```python
from build123d import *

# Parameters (mm, degrees)
SKETCH1_R                = 41.9034
SKETCH1_R_2              = 39.9034
BOSS_EXTRUDE1_DEPTH      = 57.15
BOSS_EXTRUDE2_REACH      = 137.075
BOSS_EXTRUDE2_END_RADIUS = 41.9034
SKETCH4_W                = 6.35
SKETCH4_H                = 96.707907256
CUT_EXTRUDE1_REACH       = 161.401
CUT_EXTRUDE1_END_RADIUS  = 39.9034
SKETCH5_W                = 3.2385
SKETCH5_H                = 67.115737741
CIRPATTERN1_COUNT        = 4
SKETCH6_W                = 191.094400596
SKETCH6_H                = 76.2
SKETCH6_H_2              = 57.15
CUT_EXTRUDE2_DEPTH       = 154.043134259
CUT_EXTRUDE2_DEPTH_BACK  = 154.043134259


with BuildPart() as part:
    # Sketch1 → Boss-Extrude1 (new, symmetric)
    with BuildSketch(Plane(origin=(0, 0, 0), x_dir=(1, 0, 0), z_dir=(0, 1, 0))):
        with Locations(Location((0, 0, 0), (0, 0, 270))):
            Circle(SKETCH1_R)
        with Locations(Location((0, 0, 0), (0, 0, 270))):
            Circle(SKETCH1_R_2, mode=Mode.SUBTRACT)
    extrude(amount=BOSS_EXTRUDE1_DEPTH, both=True)

    # Boss-Extrude2: up to this cylinder (the profile starts outside it)
    boss_extrude2_end = Plane(origin=(0, -4.217047, 0), z_dir=(0, -1, 0)) * Cylinder(BOSS_EXTRUDE2_END_RADIUS, 358.9568, mode=Mode.PRIVATE)
    # Sketch4 → Boss-Extrude2 (add, up to the surface)
    with BuildSketch(Plane(origin=(0, -33.016886495, -49.525456207), x_dir=(1, 0, 0), z_dir=(0, 0.5546992156114063, 0.8320509480795575)), mode=Mode.PRIVATE) as boss_extrude2_sk1:
        with Locations((0, 34.613072097)):
            Rectangle(SKETCH4_W, SKETCH4_H)
    boss_extrude2_tool1 = extrude(boss_extrude2_sk1.sketch, amount=BOSS_EXTRUDE2_REACH, mode=Mode.PRIVATE) - boss_extrude2_end
    boss_extrude2 = boss_extrude2_tool1.solids().sort_by_distance((0, -4.217047, -68.7253))[0]
    add(boss_extrude2)

    # Cut-Extrude1: up to this cylinder (the profile starts outside it)
    cut_extrude1_end = Plane(origin=(0, 56.039365, 0), z_dir=(0, -1, 0)) * Cylinder(CUT_EXTRUDE1_END_RADIUS, 403.6088, mode=Mode.PRIVATE)
    # Sketch5 → Cut-Extrude1 (cut, up to the surface)
    with BuildSketch(Plane(origin=(0, 69.032792414, -46.021744091), x_dir=(1, 0, 0), z_dir=(0, 0.8320509480795577, -0.5546992156114063)), mode=Mode.PRIVATE) as cut_extrude1_sk1:
        with Locations((0, 23.424274962)):
            Rectangle(SKETCH5_W, SKETCH5_H)
    cut_extrude1_tool1 = extrude(cut_extrude1_sk1.sketch, amount=-CUT_EXTRUDE1_REACH, mode=Mode.PRIVATE) - cut_extrude1_end
    cut_extrude1 = cut_extrude1_tool1.solids().sort_by_distance((0, 56.039365, -65.511934))[0]
    add(cut_extrude1, mode=Mode.SUBTRACT)

    # CirPattern1: Boss-Extrude2, Cut-Extrude1 ×4 about axis
    cirpattern1_axis = Axis((0, 0, 0), (0, 1, 0))
    add([boss_extrude2.rotate(cirpattern1_axis, i * 360 / CIRPATTERN1_COUNT) for i in range(1, CIRPATTERN1_COUNT)])
    add([cut_extrude1.rotate(cirpattern1_axis, i * 360 / CIRPATTERN1_COUNT) for i in range(1, CIRPATTERN1_COUNT)], mode=Mode.SUBTRACT)

    # Sketch6 → Cut-Extrude2 (cut, two sides)
    with BuildSketch(Plane(origin=(0, 0, 0), x_dir=(0, 0, -1), z_dir=(1, 0, 0))) as cut_extrude2_sk:
        with Locations((0, 33.758652745)):
            Rectangle(SKETCH6_W, SKETCH6_H)
        with Locations((0, -51.966347255)):
            Rectangle(SKETCH6_W, SKETCH6_H_2)
    extrude(amount=CUT_EXTRUDE2_DEPTH, mode=Mode.SUBTRACT)
    extrude(cut_extrude2_sk.sketch, amount=-CUT_EXTRUDE2_DEPTH_BACK, mode=Mode.SUBTRACT)


solid = part.part
```
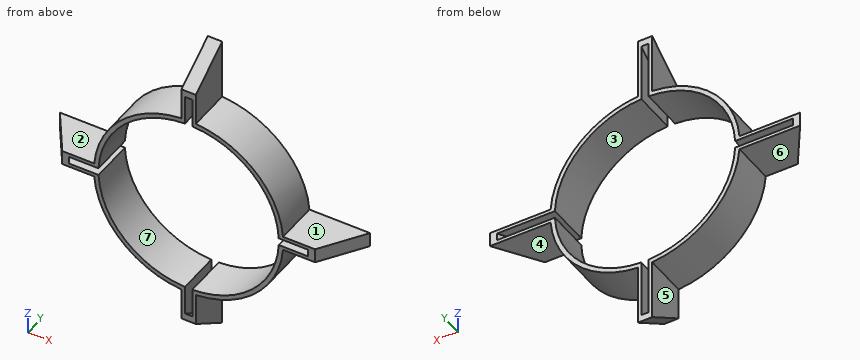
Verification items for the finished model (mm, model axes). Face numbers are marked on the shaded views. A direction names the side the tool comes from. Give positions to 0.01 mm unless a question says otherwise; leave off trailing zeros. Order: outer loops, then holes, each group sorted by start corner. A loop starts at its lowest first (then second) coordinate and runs counter-clockwise, first axis right, second up. Notation, with made-up numbers: (-21, 58) -> (-14, 58) arc R24 ccw to (-14, 85) -> close; hole circle Ø4 at (20, -1). An arc over 180 degrees is marked (long way). Use a Markdown table: item, result.
1) Section check A-A, the plane x = 12. Record the boundary of the cut face in (y, z).
Results:
| item | result |
|---|---|
| outline | (-23.39, -40.15) -> (-4.34, -40.15) -> (-4.34, -38.06) -> (-23.39, -38.06) -> close; (-23.39, 38.06) -> (-4.34, 38.06) -> (-4.34, 40.15) -> (-23.39, 40.15) -> close |
2) Section check B-B, the plane z = 16. Record the boundary of the cut face in (x, y), then the cut area to 3 significant figures.
Results:
| item | result |
|---|---|
| outline | (-38.73, -23.39) -> (-36.56, -23.39) -> (-36.56, -4.34) -> (-38.73, -4.34) -> close; (36.56, -23.39) -> (38.73, -23.39) -> (38.73, -4.34) -> (36.56, -4.34) -> close |
| area | 82.8 mm² |
3) Depth check by flat-ended pin: pin 1 Ø6 at (y, z) = (-20, -21) entering from -X; pin 2 Ø6 at (y, z) = (-20.5, 46) entering from -X (3 decimals); pin 3 Ø9.5 at (x, y) = (47, -18.5) entering from +Z (3 decimals). Enter the tip coordinate at first touch or a pass-through.
Results:
| item | result |
|---|---|
| pin 1 | x = -37.84 |
| pin 2 | x = -3.175 |
| pin 3 | z = 3.175 |
4) Mould release check, pull along X, two halves, no side actions. Record for the marked faces 5, 6 and 7: pulls with the +X half, pulls with the -X half, needs draft (parallel to the pull), parting line crosses it, or undercut.
Results:
| item | result |
|---|---|
| face 5 | pulls with the -X half |
| face 6 | needs draft |
| face 7 | undercut |
5) Tool access check on the marked faces 1, 2, 3 and 4. Record the directions out of +Z, -Z, +X, -X, +Y, -Y that give a thin tool (end or side, any length) a straight path to the whole face; none if there is none.
Results:
| item | result |
|---|---|
| face 1 | +Z, +X, +Y, -Y |
| face 2 | +Z, -X, +Y, -Y |
| face 3 | +Y, -Y |
| face 4 | -Z, +X, +Y, -Y |
6) Material ranges on probe 1 along Z at (x, y) = (56, -17) (3 decimals); probe 2 along X at (y, z) = (-17.75, -13), recorded low to high.
Results:
| item | result |
|---|---|
| probe 1 | -3.175 to -1.619, 1.619 to 3.175 |
| probe 2 | -39.84 to -37.73, 37.73 to 39.84 |
